Can you work these out from the model? Positions are in its coordinate system, mm. Face numbers are marked on the shaded views. A direction names the side the tool comes from. Give positions to 0.01 mm unless a question says otherwise; leave off trailing zeros. Loops run counter-clockwise (first coordinate to the right, second up) from the corner with the lowest first, then second, coordinate; pieces in that order, holes last. Notation, with made-up numbers: (39.25, -20) - (44.25, -20) arc R13 ccw to (44.25, 0) - close; hole circle Ø2 at (57, 35.25). An arc over 180 degrees is marked (long way). Answer in a Markdown table with one row per item.
from build123d import *

# Parameters (mm, degrees)
F0_W     = 105
F0_H     = 26
F2_DEPTH = 13
F3_DEPTH = 13
F4_DEPTH = 13
F5_DEPTH = 13
F6_SIZE  = 2.7
F7_SIZE  = 2.7


with BuildPart() as f1:
    # F0 (on Top) → F1 (revolve)
    with BuildSketch(Plane.XY):
        with BuildLine():
            Line((110, 0), (0, 0))
            Line((0, 0), (0, -10.0923664868))
            add(Edge.make_bspline(
                [(0, -10.0923664868), (8.6124591201, -9.6848175395), (24.3863467012, -8.9383836594), (36.054630575, -11.7317822521), (41.3520932198, -13)],
                knots=[0, 0, 0, 0, 0.5459947065, 1, 1, 1, 1], degree=3))
            Line((41.3520932198, -13), (106.8001613021, -13))
            ThreePointArc((106.8001613021, -13), (109.0781586072, -11.1114138074), (110, -8.2996104758))
            Line((110, -8.2996104758), (110, -7.9163433984))
            Line((110, -7.9163433984), (110, 0))
        make_face()
    revolve(axis=Axis((55, 0, 0), (1, 0, 0)))



with BuildPart() as f2:
    # F0 (on Top) → F2 (new body)
    with BuildSketch(Plane.XY):
        with Locations((-57.5, 0)):
            Rectangle(F0_W, F0_H)
    extrude(amount=F2_DEPTH)

    # F3 (add): a face of the model
    f3_faces = [f2.faces().sort_by_distance(p)[0] for p in [
        (-57.5, 0, 0),
    ]]
    extrude(f3_faces, amount=F3_DEPTH)


with BuildPart() as f4:
    # F0 (on Top) → F4 (new body)
    with BuildSketch(Plane.XY):
        Polygon((0, 0), (0, 10.0923664868), (-5, 13), (-5, -13), (0, -10.0923664868), align=None)
    extrude(amount=F4_DEPTH)


with BuildPart() as f1_1:
    add(f1.part)
    # F5 (add): a face of the model
    f5_faces = [f4.part.faces().sort_by_distance(p)[0] for p in [
        (-2.6049276578, 0, 0),
    ]]

    add(f2.part)  # F5 merges F2

    add(f4.part)  # F5 merges F4
    extrude(f5_faces, amount=F5_DEPTH)

    # F6
    f6_edges = [f1_1.edges().sort_by_distance(p)[0] for p in [
        (0, 0, 13),
    ]]
    chamfer(f6_edges, length=F6_SIZE)

    # F7
    f7_edges = [f1_1.edges().sort_by_distance(p)[0] for p in [
        (0, 0, -13),
    ]]
    chamfer(f7_edges, length=F7_SIZE)


solid = f1_1.part
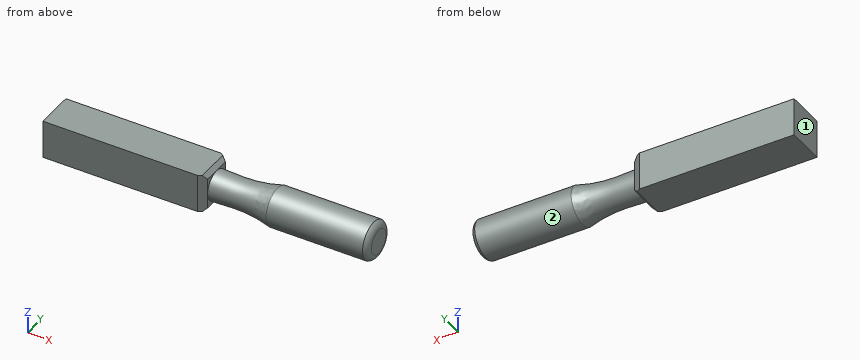
Q1. On a 3-axis mill with a long thin cutter (end or side, diameter ignored), from which of +Z, -Z, +X, -X, +Y, -Y can I reach the whole of each face in a straight line? I mean the marked faces 1 and 2. Say none if no direction works.
Checked values:
| item | result |
|---|---|
| face 1 | +Z, -Z, -X, +Y, -Y |
| face 2 | +X |
Q2. Imagine slicing it at A-A, the plane x = 75. Write out the boundary of the cut face in (y, z), and give its area (3 significant figures).
Checked values:
| item | result |
|---|---|
| outline | circle Ø26 at (0, 0) |
| area | 531 mm² |
Q3. For pin 1 (2 mm diameter, centred on y = 4.5, z = -9, fed in from +X); pin 2 (1.5 mm diameter, centred on x = 64, z = 3.5, fed in from +Y); pin 3 (6 mm diameter, centred on y = 7, z = 10.5, fed in from +X), each with a flat end and sliding along its axis, tell me the tip position at first contact or that it passes through.
Checked values:
| item | result |
|---|---|
| pin 1 | stops at x = 109.92 |
| pin 2 | stops at y = 12.71 |
| pin 3 | stops at x = 109.78 |
Q4. If I drill on line 1 (X direction, y = -4.5, z = -7); line 2 (Y direction, x = 74.5, z = -5.5); line 3 (Y direction, x = 100, z = -6), over which ranges is the centre line in solid material (lowest first)? Write a range as [from, to].
Checked values:
| item | result |
|---|---|
| line 1 | x = [-110, 110] |
| line 2 | y = [-11.78, 11.78] |
| line 3 | y = [-11.53, 11.53] |
